Source: CAD feature listing. Evaluate the final solid. Frame: model axes, mm. Coordinates: 2 decimals unless noted, no trailing zeros. Loops run counter-clockwise (first coordinate to the right, second up) from the corner with the lowest first, then second, coordinate; pieces in that order, holes last. Notation, with made-up numbers: (53, 7.25) -> (70, 7.25) arc R29 cw to (70, 32.25) -> close; hole circle Ø4 at (47.5, 70.25). An arc over 180 degrees is marked (long way). Answer as a JSON object with one key per item and string values. Group by question number.
from build123d import *

# Parameters (mm, degrees)
SKETCH1_R           = 2.5
BOSS_EXTRUDE1_DEPTH = 20
FILLET1_R           = 5


with BuildPart() as part:
    # Sketch1 → Boss-Extrude1 (new body)
    with BuildSketch(Plane(origin=(0, 0, 0), x_dir=(1, 0, 0), z_dir=(0, 1, 0))):
        with BuildLine():
            Line((0, 30), (0, 5))
            ThreePointArc((0, 5), (3.535533906, -3.535533906), (-5, 0))
            Line((-5, 0), (-5, 5))
            Line((-5, 5), (-5, 30))
            Line((-5, 30), (0, 30))
        make_face()
        with Locations(Location((0, 0, 0), (0, 0, 270))):
            Circle(SKETCH1_R, mode=Mode.SUBTRACT)
    extrude(amount=BOSS_EXTRUDE1_DEPTH)

    # Fillet1
    fillet1_edges = [part.edges().sort_by_distance(p)[0] for p in [
        (-5, 10, -30),
    ]]
    fillet(fillet1_edges, radius=FILLET1_R - 0.0001)  # a hair under: the kernel refuses the full size


solid = part.part
1. Section query C-C on z = -25.5. Return loops of the section in (x, y), then the cut area to 3 significant figures.
2. Ray query, L1, parallel to X at y = 13.5, z = -6.5; L2, parallel to Z at x = -0.75, y = 15.25; L3, parallel to Z at x = 2, y = 19.25. Return the intervals inside material, ascending.
3. Pin query (flat end, axial travel): pin 1 Ø4 at (x, y) = (3.5, 17.5) entering from +Z; pin 2 Ø6 at (y, z) = (15, -23.5) entering from +X; pin 3 Ø1.5 at (x, y) = (3.5, 17.5) entering from +Z. Return the tip coordinate at first contact, or that it passes through.
4. Mould query, pull axis X, two halves, no side actions, for faces 1 (the face through (0, 10, -18)), 2 (the face through (-2.44, 9.86, -0.54)), 3 (the face through (-5, 10, -12)). Classes: pulls with the +X half, pulls with the -X half, needs draft (parallel to the pull), parting line crosses it, or undercut.
5. Section query B-B on z = -19.5. Return loops of the section in (x, y).
Solved:
{
 "1": {"outline": "(-4.97, 0) -> (0, 0) -> (0, 20) -> (-4.97, 20) -> close", "area": "99.5 mm^2"},
 "2": {"L1": "-5 to 0", "L2": "-29.94 to -2.38, 2.38 to 4.94", "L3": "-4.58 to -1.5, 1.5 to 4.58"},
 "3": {"pin 1": "z = 4.77", "pin 2": "x = 0", "pin 3": "z = 4.18"},
 "4": {"face 1": "pulls with the +X half", "face 2": "undercut", "face 3": "pulls with the -X half"},
 "5": {"outline": "(-5, 0) -> (0, 0) -> (0, 20) -> (-5, 20) -> close"}
}
